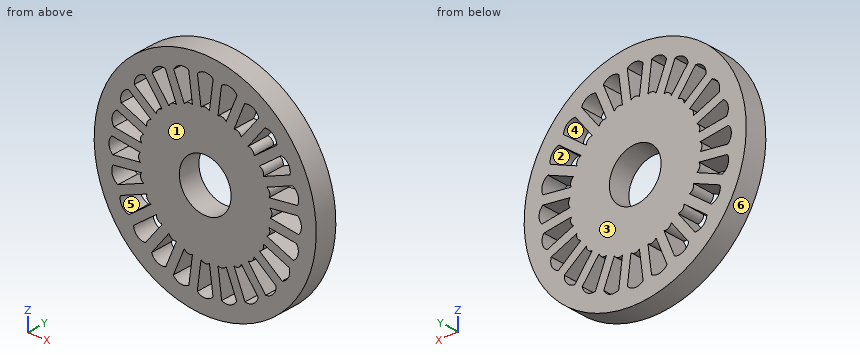
from build123d import *

# Parameters (mm, degrees)
SKETCH2_R           = 12.875
SKETCH2_R_2         = 3
BOSS_EXTRUDE1_DEPTH = 2.55
CUT_EXTRUDE1_DEPTH  = 2.55
CIRPATTERN1_COUNT   = 24


with BuildPart() as part:
    # Sketch2 → Boss-Extrude1 (new body)
    with BuildSketch(Plane(origin=(0, 0, 0), x_dir=(1, 0, 0), z_dir=(0, 1, 0))):
        with Locations(Location((0, 0, 0), (0, 0, 270))):
            Circle(SKETCH2_R)
        with Locations(Location((0, 0, 0), (0, 0, 270))):
            Circle(SKETCH2_R_2, mode=Mode.SUBTRACT)
    extrude(amount=BOSS_EXTRUDE1_DEPTH)

    # Sketch4 → Cut-Extrude1 (cut)
    with BuildSketch(Plane(origin=(0, 2.55, 0), x_dir=(1, 0, 0), z_dir=(0, 1, 0))):
        with BuildLine():
            Line((0.486824592, 7.528448687), (0.906471755, 10.715985352))
            ThreePointArc((0.906471755, 10.715985352), (0.015796353, 11.15041104), (-0.921191613, 10.827793773))
            Line((-0.921191613, 10.827793773), (-0.486824592, 7.528448687))
            ThreePointArc((-0.486824592, 7.528448687), (0, 7.730098035), (0.486824592, 7.528448687))
        make_face()
    cut_extrude1 = extrude(amount=-CUT_EXTRUDE1_DEPTH, mode=Mode.SUBTRACT)

    # CirPattern1: Cut-Extrude1 ×24 about axis
    cirpattern1_axis = Axis((0, 0, 0), (0, 1, 0))
    for i in range(1, CIRPATTERN1_COUNT):
        add(cut_extrude1.rotate(cirpattern1_axis, i * 360 / CIRPATTERN1_COUNT), mode=Mode.SUBTRACT)


solid = part.part
Verification items for the finished model (mm, model axes). Face numbers are marked on the shaded views. A direction names the side the tool comes from. Coordinates: 2 decimals unless noted, no trailing zeros. Loops run counter-clockwise (first coordinate to the right, second up) from the corner with the lowest first, then second, coordinate; pieces in that order, holes last. Notation, with made-up numbers: M 44,89 L 65,89 A38 ccw 65,128 Z; hole C -11.5,-0.5 d1. An arc over 180 degrees is marked long. One line per item, written item: value.
1. Material ranges on line 1 along X through (y, z) = (1.2, 0) (3 decimals); line 2 along X through (y, z) = (2.25, 4.5); line 3 along Z through (x, y) = (8.5, 1.65), recorded low to high. Write a range as from..to.
Answers follow:
line 1: -12.875..-11.151, -7.73..-3, 3..7.73, 11.151..12.875
line 2: -12.06..-9.56, -6.69..6.69, 9.56..12.06
line 3: -9.67..-5.89, -4.06..-2.98, -1.62..-0.61, 0.61..1.62, 2.98..4.06, 5.89..9.67
2. Gauge pin test, flat ends, axial feed: P1, Ø5, axis at x = 0, z = 0, coming from the +Y side; P2, Ø1.5, axis at y = 1.5, z = 6, coming from the -X side; P3, Ø1.5, axis at y = 1.5, z = -1, coming from the +X side; P4, Ø1.5, axis at y = 1, z = -7, coming from the +X side. Record the tip position at first contact, or that the pin passes through.
Answers follow:
P1: through
P2: x = -11.76
P3: x = 12.87
P4: x = 11.26
3. Section check A-A on z = 0. Record the cut outline in (x, y) (3 decimals).
Answers follow:
outline: M -12.875,0 L -11.151,0 L -11.151,2.55 L -12.875,2.55 Z; M -7.73,0 L -3,0 L -3,2.55 L -7.73,2.55 Z; M 3,0 L 7.73,0 L 7.73,2.55 L 3,2.55 Z; M 11.151,0 L 12.875,0 L 12.875,2.55 L 11.151,2.55 Z
4. Section check C-C on y = 1.25. Give the number of separate pieces and of enclosed holes in the cut face, plus the area to 3 significant figures.
Answers follow:
separate pieces: 1
enclosed holes: 25
area: 375 mm^2
5. Section check B-B on x = 0. Record the cut outline in (y, z) (3 decimals), plus the area to 3 significant figures.
Answers follow:
outline: M 0,-12.875 L 2.55,-12.875 L 2.55,-11.151 L 0,-11.151 Z; M 0,-7.73 L 2.55,-7.73 L 2.55,-3 L 0,-3 Z; M 0,3 L 2.55,3 L 2.55,7.73 L 0,7.73 Z; M 0,11.151 L 2.55,11.151 L 2.55,12.875 L 0,12.875 Z
area: 32.9 mm^2
6. Set-up check for the marked faces 1 and 2: record each of +Z, -Z, +X, -X, +Y, -Y from which the full face is reachable in a straight line by a thin tool's end or side.
Answers follow:
face 1: +Z, -Z, +X, -X, -Y
face 2: +Y, -Y
7. Mould release check, pull along X, two halves, no side actions. Record for the marked faces 3, 4, 5 and 6: pulls with the +X half, pulls with the -X half, needs draft (parallel to the pull), parting line crosses it, or undercut.
Answers follow:
face 3: needs draft
face 4: undercut
face 5: undercut
face 6: parting line crosses it
